Input: part model. Units: mm. Frame: model coordinates. Face numbers are marked on the shaded views. A direction names the side the tool comes from. Coordinates: 2 decimals unless noted, no trailing zeros. Order: outer loops, then holes, each group sorted by start corner. A loop starts at its lowest first (then second) coordinate and runs counter-clockwise, first axis right, second up. Notation, with made-up numbers: (-27.75, 53.5) -> (-18.75, 53.5) arc R16 cw to (-18.75, 77.5) -> close; hole circle Ø11 at (-19.5, 38.5). An arc over 180 degrees is marked (long way). Answer as CSV lines item,"result".
from build123d import *

# Parameters (mm, degrees)
BOSS_EXTRUDE1_DEPTH  = 2.54
SKETCH2_W            = 3.048
SKETCH2_H            = 25.4
BOSS_EXTRUDE2_DEPTH  = 12.7
FILLET5_R            = 12.7
FILLET6_R            = 12.7
FILLET7_R            = 12.7
FILLET8_R            = 12.7
SKETCH3_R            = 1.5875
CUT_EXTRUDE1_DEPTH   = 187.084255379
SKETCH4_W            = 12.7
SKETCH4_H            = 12.7
SKETCH4_R            = 1.5875
BOSS_EXTRUDE3_DEPTH  = 3.175
BOSS_EXTRUDE4_DEPTH  = 6.35
FILLET10_R           = 6.35
FILLET11_R           = 6.35
SKETCH6_W            = 3.175
SKETCH6_H            = 19.05
CUT_EXTRUDE2_DEPTH   = 3.175
BOSS_EXTRUDE5_DEPTH  = 25.4
FILLET12_R           = 25.4
SKETCH8_W            = 133.35
SKETCH8_H            = 3.175
BOSS_EXTRUDE6_DEPTH  = 25.4
BOSS_EXTRUDE9_DEPTH  = 114.554
CUT_EXTRUDE3_REACH   = 177.181
BOSS_EXTRUDE10_DEPTH = 12.7
BOSS_EXTRUDE11_DEPTH = 12.7
CUT_EXTRUDE4_DEPTH   = 185.822136131
FILLET15_R           = 101.6
SKETCH14_R           = 1.5875
BOSS_EXTRUDE12_DEPTH = 3.175


# Some blends are built 0.0001 mm under size
with BuildPart() as part:
    # Sketch1 → Boss-Extrude1 (new body)
    with BuildSketch(Plane(origin=(0, 0, 0), x_dir=(1, 0, 0), z_dir=(0, 1, 0))):
        Polygon((15.748, -114.3), (130.302, -114.3), (130.302, -88.9), (143.002, -88.9), (143.002, -114.3), (146.05, -114.3), (146.05, 0), (0, 0), (0, -114.3), (3.048, -114.3), (3.048, -88.9), (15.748, -88.9), align=None)
    extrude(amount=BOSS_EXTRUDE1_DEPTH)

    # Sketch2 → Boss-Extrude2 (add)
    with BuildSketch(Plane(origin=(0, 2.54, 0), x_dir=(1, 0, 0), z_dir=(0, 1, 0))):
        with Locations((1.524, -101.6)):
            Rectangle(SKETCH2_W, SKETCH2_H)
    boss_extrude2 = extrude(amount=BOSS_EXTRUDE2_DEPTH)

    # Mirror1: Boss-Extrude2 across plane
    add(boss_extrude2.mirror(Plane(origin=(73.025, 0, 0), x_dir=(0, 0, 1), z_dir=(1, 0, 0))))

    # Fillet5
    fillet5_edges = [part.edges().sort_by_distance(p)[0] for p in [
        (1.524, 15.24, 114.3),
        (1.524, 15.24, 88.9),
    ]]
    fillet(fillet5_edges, radius=FILLET5_R - 0.0001)  # a hair under: the kernel refuses the full size

    # Fillet6
    # the kernel refuses this fillet: 12.7 mm, written as the material it adds along each edge
    with BuildSketch(Plane(origin=(3.048, 2.54, 88.9), x_dir=(0, 0.9659271393953295, 0.25881414447351125), z_dir=(-1, 0, 0))) as fillet6_piece_1:
        with BuildLine():
            CenterArc((9.861056917, 12.267248789), FILLET6_R, 194.99970931, 60.000130236)
            Line((-2.406217753, 8.980309154), (-3.63294522, 8.65161519))
            Line((-3.63294522, 8.65161519), (-1.226727467, -0.328693963))
            Line((-1.226727467, -0.328693963), (0.328693963, -1.226727467))
            ThreePointArc((0.328693963, -1.226727467), (0.328790556, -1.226701586), (6.245317068, -1.226724879))
            Line((6.245317068, -1.226724879), (6.574020691, 0))
        make_face()
    extrude(amount=3.048)

    # Fillet7
    fillet7_edges = [part.edges().sort_by_distance(p)[0] for p in [
        (144.526, 15.24, 88.9),
        (144.526, 15.24, 114.3),
    ]]
    fillet(fillet7_edges, radius=FILLET7_R - 0.0001)  # a hair under: the kernel refuses the full size

    # Fillet8
    # the kernel refuses this fillet: 12.7 mm, written as the material it adds along each edge
    with BuildSketch(Plane(origin=(143.002, 2.54, 88.9), x_dir=(0, 0, -1), z_dir=(1, 0, 0))) as fillet8_piece_1:
        with BuildLine():
            CenterArc((9.297087521, 12.7), FILLET8_R, 209.999869764, 60.000130236)
            Line((-1.701449541, 6.350025), (-2.801303247, 5.7150275))
            ThreePointArc((-2.801303247, 5.7150275), (-1.27, 0.0001), (-1.27, 0))
            Line((-1.27, 0), (0, -1.27))
            Line((0, -1.27), (9.297087521, -1.27))
            Line((9.297087521, -1.27), (9.297087521, 0))
        make_face()
    extrude(amount=3.048)

    # Sketch3 → Cut-Extrude1 (cut, through all)
    with BuildSketch(Plane(origin=(146.05, 0, 0), x_dir=(0, 0, -1), z_dir=(1, 0, 0))):
        with Locations((-101.6, 7.935875783)):
            Circle(SKETCH3_R)
    extrude(amount=-CUT_EXTRUDE1_DEPTH, mode=Mode.SUBTRACT)

    # Sketch4 → Boss-Extrude3 (add)
    with BuildSketch(Plane(origin=(146.05, 0, 0), x_dir=(0, 0, -1), z_dir=(1, 0, 0))):
        with Locations((0, 8.89)):
            Rectangle(SKETCH4_W, SKETCH4_H)
        with Locations((0, 7.935875783)):
            Circle(SKETCH4_R, mode=Mode.SUBTRACT)
    boss_extrude3 = extrude(amount=-BOSS_EXTRUDE3_DEPTH)

    # Sketch5 → Boss-Extrude4 (add)
    with BuildSketch(Plane(origin=(0, 0, 0), x_dir=(-1, 0, 0), z_dir=(0, 0, -1))):
        Polygon((-146.05, 0), (0, 0), (0, 2.54), (-142.875, 2.54), (-146.05, 2.54), align=None)
    extrude(amount=BOSS_EXTRUDE4_DEPTH)

    # Mirror2: Boss-Extrude3 across plane
    add(boss_extrude3.mirror(Plane(origin=(73.025, 0, 0), x_dir=(0, 0, 1), z_dir=(1, 0, 0))))

    # Fillet10
    fillet10_edges = [part.edges().sort_by_distance(p)[0] for p in [
        (1.5875, 15.24, 6.35),
        (1.5875, 15.24, -6.35),
        (144.4625, 15.24, -6.35),
        (144.4625, 15.24, 6.35),
    ]]
    fillet(fillet10_edges, radius=FILLET10_R - 0.0001)  # a hair under: the kernel refuses the full size

    # Fillet11
    fillet11_edges = [part.edges().sort_by_distance(p)[0] for p in [
        (1.5875, 2.54, 6.35),
        (144.4625, 2.54, 6.35),
    ]]
    fillet(fillet11_edges, radius=FILLET11_R)

    # Sketch6 → Cut-Extrude2 (cut)
    with BuildSketch(Plane.XZ):
        with Locations((141.2875, 3.175)):
            Rectangle(SKETCH6_W, SKETCH6_H)
    cut_extrude2 = extrude(amount=-CUT_EXTRUDE2_DEPTH, mode=Mode.SUBTRACT)

    # Mirror3: Cut-Extrude2 across plane
    add(cut_extrude2.mirror(Plane(origin=(73.025, 0, 0), x_dir=(0, 0, 1), z_dir=(1, 0, 0))), mode=Mode.SUBTRACT)

    # Sketch7 → Boss-Extrude5 (add)
    with BuildSketch(Plane.XZ):
        Polygon((143.002, 114.3), (146.05, 114.3), (146.05, -6.35), (142.875, -6.35), (142.875, 12.7), (143.002, 88.9), align=None)
    boss_extrude5 = extrude(amount=BOSS_EXTRUDE5_DEPTH)

    # Mirror4: Boss-Extrude5 across plane
    add(boss_extrude5.mirror(Plane(origin=(73.025, 0, 0), x_dir=(0, 0, 1), z_dir=(1, 0, 0))))

    # Fillet12
    fillet12_edges = [part.edges().sort_by_distance(p)[0] for p in [
        (1.524, -25.4, 114.3),
        (144.526, -25.4, 114.3),
    ]]
    fillet(fillet12_edges, radius=FILLET12_R)

    # Sketch8 → Boss-Extrude6 (add)
    with BuildSketch(Plane.XZ):
        with Locations((73.025, -4.7625)):
            Rectangle(SKETCH8_W, SKETCH8_H)
    extrude(amount=BOSS_EXTRUDE6_DEPTH)

    # Sketch9 → Boss-Extrude9 (add)
    with BuildSketch(Plane.ZY.offset(-15.748)):
        Polygon((114.3, -9.24484395), (114.3, -7.643590007), (93.299409051, 0), (88.9, 0), align=None)
    extrude(amount=-BOSS_EXTRUDE9_DEPTH)

    # Sketch10 → Cut-Extrude3 (cut, up to next)
    with BuildSketch(Plane.ZY.offset(-15.748), mode=Mode.PRIVATE) as cut_extrude3_sk1:
        Polygon((93.299409051, 0), (88.9, 2.54), (114.3, 2.54), (114.3, 0), align=None)
    cut_extrude3_tool1 = extrude(cut_extrude3_sk1.sketch, amount=-CUT_EXTRUDE3_REACH, mode=Mode.PRIVATE) & part.part
    add(cut_extrude3_tool1.solids().sort_by_distance((15.748, 1.310138, 102.665092))[0], mode=Mode.SUBTRACT)

    # Sketch11 → Boss-Extrude10 (add)
    with BuildSketch(Plane.ZY.offset(-15.748)):
        Polygon((114.3, -7.643590007), (93.299409051, 0), (88.9, 2.54), (88.9, 0), (114.3, -9.24484395), align=None)
    extrude(amount=BOSS_EXTRUDE10_DEPTH)

    # Sketch12 → Boss-Extrude11 (add)
    with BuildSketch(Plane(origin=(130.302, 0, 0), x_dir=(0, 0, -1), z_dir=(1, 0, 0))):
        Polygon((-88.9, 0), (-88.9, 2.54), (-93.299409051, 0), (-114.3, -7.643590007), (-114.3, -9.24484395), align=None)
    extrude(amount=BOSS_EXTRUDE11_DEPTH)

    # Sketch13 → Cut-Extrude4 (cut, through all)
    with BuildSketch(Plane.ZY.offset(-3.048)):
        with BuildLine():
            Line((114.3, -7.643590007), (113.240908135, -7.258112093))
            ThreePointArc((113.240908135, -7.258112093), (113.015140482, -7.976214611), (112.768192568, -8.68731164))
            Line((112.768192568, -8.68731164), (114.3, -9.24484395))
            Line((114.3, -9.24484395), (114.3, -7.643590007))
        make_face()
    extrude(amount=-CUT_EXTRUDE4_DEPTH, mode=Mode.SUBTRACT)

    # Fillet15
    fillet15_edges = [part.edges().sort_by_distance(p)[0] for p in [
        (73.025, 0, 88.9),
    ]]
    fillet(fillet15_edges, radius=FILLET15_R)

    # Sketch14 → Boss-Extrude12 (add)
    with BuildSketch(Plane.ZY.offset(-6.35)):
        with BuildLine():
            Line((-6.35, 2.54), (12.7, 2.54))
            ThreePointArc((12.7, 2.54), (8.209871939, 4.399871939), (6.35, 8.89))
            ThreePointArc((6.35, 8.89), (4.490128061, 13.380128061), (0, 15.24))
            ThreePointArc((0, 15.24), (-4.490128061, 13.380128061), (-6.35, 8.89))
            Line((-6.35, 8.89), (-6.35, 2.54))
        make_face()
        with Locations(Location((0, 7.935875783, 0), (0, 0, 180))):
            Circle(SKETCH14_R, mode=Mode.SUBTRACT)
    boss_extrude12 = extrude(amount=-BOSS_EXTRUDE12_DEPTH)

    # Mirror5: Boss-Extrude12 across plane
    add(boss_extrude12.mirror(Plane(origin=(73.025, 0, 0), x_dir=(0, 0, 1), z_dir=(1, 0, 0))))


solid = part.part
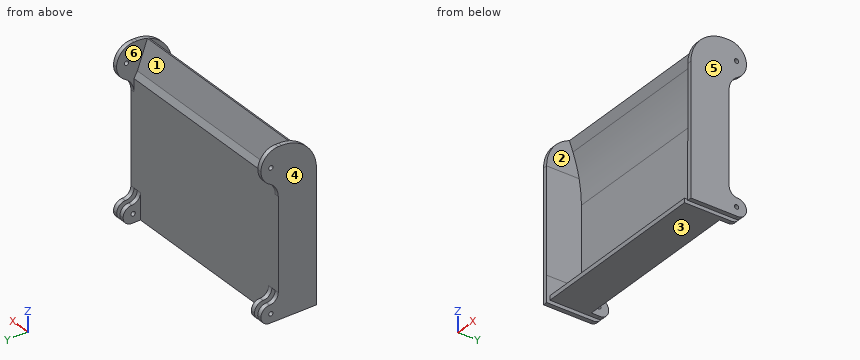
1. Cut plane A-A (y = -17). Return the cut outline in (x, z) (3 decimals), plus the area to 3 significant figures.
Findings:
outline,"(0, -6.35) -> (3.175, -6.35) -> (3.175, 12.7) -> (3.048, 88.9) -> (3.048, 107.772) -> (0, 107.772) -> close; (6.35, -6.35) -> (139.7, -6.35) -> (139.7, -3.175) -> (6.35, -3.175) -> close; (142.875, -6.35) -> (146.05, -6.35) -> (146.05, 107.772) -> (143.002, 107.772) -> (143.002, 88.9) -> (142.875, 12.7) -> close"
area,"1,130 mm2"
2. Cut plane D-D (z = 58.5). Return the cut outline in (x, y), plus the area to 3 significant figures.
Findings:
outline,"(0, -25.4) -> (3.1, -25.4) -> (3.1, 0) -> (142.95, 0) -> (142.95, -25.4) -> (146.05, -25.4) -> (146.05, 2.54) -> (0, 2.54) -> close"
area,"528 mm2"
3. Contact query for flat-ended pins moving along their axis: pin 1 (3 mm diameter, centred on y = -18, z = 70, fed in from -X); pin 2 (8 mm diameter, centred on x = 23, z = 82.5, fed in from +Y); pin 3 (12.5 mm diameter, centred on x = 84, y = -14.5, fed in from +Z); pin 4 (3 mm diameter, centred on y = 7.94, z = 0, fed in from -X). Output: stop coordinate, or through.
Findings:
pin 1,"stops at x = 0"
pin 2,"stops at y = 2.54"
pin 3,"stops at z = 112.92"
pin 4,"passes through"
4. Cut plane C-C (x = 24.5). Return the cut outline in (y, z) (3 decimals), plus the area to 3 significant figures.
Findings:
outline,"(-25.4, -6.35) -> (2.54, -6.35) -> (2.54, 88.9) -> (0, 93.299) -> (-7.258, 113.241) arc R25.4 ccw to (-8.687, 112.768) -> (-6.127, 105.734) arc R101.6 cw to (0, 70.985) -> (0, -3.175) -> (-25.4, -3.175) -> close"
area,"382 mm2"
5. Reachability of the marked faces 1, 2 and 3 from +Z, -Z, +X, -X, +Y, -Y: full face, straight path, thin tool, end or side. Return the list, or none.
Findings:
face 1,"+Z, +Y"
face 2,"-Y"
face 3,"-Z, +X, -X, +Y, -Y"
6. Ray query, line 1 along X through (y, z) = (-22.5, 7.5) (3 decimals); line 2 along X through (y, z) = (-3.5, 95.5); line 3 along Y through (x, z) = (144, 0). Return the intervals inside material, ascending.
Findings:
line 1,"x = 0 to 3.175, 142.875 to 146.05"
line 2,"x = 0 to 3.05, 143 to 146.05"
line 3,"y = -25.4 to 6.35, 9.52 to 15.24"
7. Cut plane B-B (z = 29.5). Return the cut outline in (x, y).
Findings:
outline,"(0, -25.4) -> (3.15, -25.4) -> (3.15, 0) -> (142.9, 0) -> (142.9, -25.4) -> (146.05, -25.4) -> (146.05, 2.54) -> (0, 2.54) -> close"
8. Mould query, pull axis X, two halves, no side actions, for the marked faces 4, 5 and 6. Classes: released by +X, released by -X, zero draft, split by the parting line, or undercut.
Findings:
face 4,"released by -X"
face 5,"released by +X"
face 6,"undercut"
